Here's how the part is built. I have some questions about the finished solid (model axes, mm). A direction names the side the tool comes from. Round coordinates to 2 decimals unless told otherwise and drop trailing zeros. Order: outer loops, then holes, each group sorted by start corner. A loop starts at its lowest first (then second) coordinate and runs counter-clockwise, first axis right, second up. Notation, with made-up numbers: (32.5, 70) -> (58.5, 70) arc R21 cw to (58.5, 76) -> close; hole circle Ø5 at (73, 82). An arc over 180 degrees is marked (long way). One line per item, written item: value.
```python
from build123d import *

# Parameters (mm, degrees)
SKETCH2_R           = 3.4
BOSS_EXTRUDE2_DEPTH = 10
SKETCH3_R           = 1.5
CUT_EXTRUDE1_DEPTH  = 30


with BuildPart() as part:
    # Sketch2 → Boss-Extrude2 (new body)
    with BuildSketch(Plane.XY):
        with BuildLine():
            Line((-3.046772292, 9.5), (3.21957788, 9.5))
            Line((3.21957788, 9.5), (17.554684003, 5.275299758))
            ThreePointArc((17.554684003, 5.275299758), (21.498894584, -0.089376976), (17.382422577, -5.32303839))
            Line((17.382422577, -5.32303839), (9, -7.5))
            Line((9, -7.5), (9, -14.5))
            Line((9, -14.5), (0.740403033, -14.5))
            Line((0.740403033, -14.5), (0.740403033, -3.930878191))
            ThreePointArc((0.740403033, -3.930878191), (0, 4), (-0.740403033, -3.930878191))
            Line((-0.740403033, -3.930878191), (-0.740403033, -14.5))
            Line((-0.740403033, -14.5), (-9, -14.5))
            Line((-9, -14.5), (-9, -7.5))
            Line((-9, -7.5), (-17.597446952, -5.249385871))
            ThreePointArc((-17.597446952, -5.249385871), (-21.499891691, 0.047111305), (-17.533036453, 5.295541242))
            Line((-17.533036453, 5.295541242), (-3.046772292, 9.5))
        make_face()
        with Locations((-15.99999429, 0.013516845)):
            Circle(SKETCH2_R, mode=Mode.SUBTRACT)
        with Locations((16, 0)):
            Circle(SKETCH2_R, mode=Mode.SUBTRACT)
    extrude(amount=BOSS_EXTRUDE2_DEPTH)

    # Sketch3 → Cut-Extrude1 (cut)
    with BuildSketch(Plane.ZY.offset(9)):
        with Locations((5, -11)):
            Circle(SKETCH3_R)
    extrude(amount=-CUT_EXTRUDE1_DEPTH, mode=Mode.SUBTRACT)


solid = part.part
```
Q1. I want a section at A-A on y = -8.5. Write out the boundary of the cut face in (x, z).
Answers:
outline: (-9, 0) -> (-0.74, 0) -> (-0.74, 10) -> (-9, 10) -> close; (0.74, 0) -> (9, 0) -> (9, 10) -> (0.74, 10) -> close
Q2. I want a section at D-D on x = 16. Write out the boundary of the cut face in (y, z).
Answers:
outline: (-5.68, 0) -> (-3.4, 0) -> (-3.4, 10) -> (-5.68, 10) -> close; (3.4, 0) -> (5.73, 0) -> (5.73, 10) -> (3.4, 10) -> close
Q3. Which directions (+Z, -Z, +X, -X, +Y, -Y) give clear straight access to the entire face, cutting with the end or side of a thin tool? Please do faces 1 (the face through (9, -9, 5)), 2 (the face through (0.74, -9, 5)), 3 (the face through (-19.397, 0.163, 4.93)).
Answers:
face 1: +Z, -Z, +X, -Y
face 2: +Z, -Z, -Y
face 3: +Z, -Z
Q4. I need wall thicknesses on line 1 along X through (y, z) = (2.5, 0.75); line 2 along X through (y, z) = (-9.5, 8.5); line 3 along X through (y, z) = (1, 2.5). Which ranges of each line are inside material? Lowest first, please.
Answers:
line 1: -20.91 to -18.32, -13.68 to -3.12, 3.12 to 13.7, 18.3 to 20.9
line 2: -9 to -0.74, 0.74 to 9
line 3: -21.41 to -19.25, -12.75 to -3.87, 3.87 to 12.75, 19.25 to 21.41
Q5. I want a section at B-B on z = 4.5. Write out the boundary of the cut face in (x, y).
Answers:
outline: (-17.6, -5.25) -> (-9, -7.5) -> (-9, -9.59) -> (-0.74, -9.59) -> (-0.74, -3.93) arc R4 cw (long way) to (0.74, -3.93) -> (0.74, -9.59) -> (9, -9.59) -> (9, -7.5) -> (17.38, -5.32) arc R5.5 ccw to (17.55, 5.28) -> (3.22, 9.5) -> (-3.05, 9.5) -> (-17.53, 5.3) arc R5.5 ccw to start; (-9, -14.5) -> (-0.74, -14.5) -> (-0.74, -12.41) -> (-9, -12.41) -> close; (0.74, -14.5) -> (9, -14.5) -> (9, -12.41) -> (0.74, -12.41) -> close; hole circle Ø6.8 at (-16, 0.01); hole circle Ø6.8 at (16, 0)
Q6. I want a section at C-C on y = -11. Write out the boundary of the cut face in (x, z), then the cut area to 3 significant figures.
Answers:
outline: (-9, 0) -> (-0.74, 0) -> (-0.74, 3.5) -> (-9, 3.5) -> close; (-9, 6.5) -> (-0.74, 6.5) -> (-0.74, 10) -> (-9, 10) -> close; (0.74, 0) -> (9, 0) -> (9, 3.5) -> (0.74, 3.5) -> close; (0.74, 6.5) -> (9, 6.5) -> (9, 10) -> (0.74, 10) -> close
area: 116 mm2
Q7. If we mould it in two halves opening along X, with no side actions, what happens to faces 4 (the face through (13.25, -6.396, 4.93)), 5 (the face through (4.81, -12.33, 5.69)), 6 (the face through (0, 4, 5)), 7 (the face through (-9, -13, 5))? For each: pulls with the +X half, pulls with the -X half, needs draft (parallel to the pull), parting line crosses it, or undercut.
Answers:
face 4: pulls with the +X half
face 5: needs draft
face 6: undercut
face 7: pulls with the -X half
Q8. For P1, Ø4, axis at x = -16, y = 0.01, coming from the +Z side; P2, Ø4, axis at y = -11, z = 5, coming from the +X side; P3, Ø5, axis at y = -4.5, z = 3.5, coming from the -X side; P4, Ø5, axis at y = -11, z = 5, coming from the -X side, each with a flat end and sliding along its axis, tell me the tip position at first contact or that it passes through.
Answers:
P1: through
P2: x = 9
P3: x = -21.12
P4: x = -9
